Verification items for the finished model (mm, model axes). Face numbers are marked on the shaded views. A direction names the side the tool comes from. Give positions to 0.01 mm unless a question says otherwise; leave off trailing zeros. Order: outer loops, then holes, each group sorted by start corner. A loop starts at its lowest first (then second) coordinate and runs counter-clockwise, first axis right, second up.
(1) Scan lines: L1, parallel to X at y = 3, z = 0; L2, parallel to X at y = 21, z = 0; L3, parallel to X at y = 2.5, z = -6.35. Record each from-to range of solid material in increasing order.
(2) Mould release check, pull along X, two halves, no side actions. Record for the marked faces 3, 4, 5 and 6: pulls with the +X half, pulls with the -X half, needs draft (parallel to the pull), parting line crosses it, or undercut.
(3) Sectioned sample at C-C on x = 0. Record the cut outline in (y, z), plus the area to 3 significant figures.
(4) Sectioned sample at A-A on y = 36.5. Count the separate pieces of the cut face and the enclosed holes in it, plus the area to 3 significant figures.
(5) Access from +Z, -Z, +X, -X, +Y, -Y to the whole of each face (thin tool, end or side, straight path). Record for the marked faces 1 and 2.
(6) Gauge pin test, flat end, axial feed: pin 1 (2 mm diameter, centred on x = -2.5, z = 15.5, fed in from +Y). Record the tip position at first contact, or that the pin passes through.
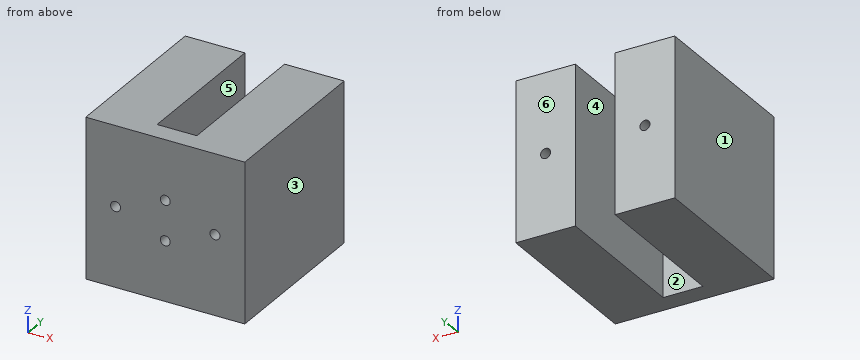
```python
from build123d import *

# Parameters (mm, degrees)
SKETCH1_W           = 50.8
SKETCH1_H           = 50.8
BOSS_EXTRUDE1_DEPTH = 6.35
SKETCH2_W           = 19.05
SKETCH2_H           = 50.8
BOSS_EXTRUDE2_DEPTH = 47.625
SKETCH3_R           = 1.5875
CUT_EXTRUDE1_DEPTH  = 60.652834174
SKETCH4_R           = 1.5875
CUT_EXTRUDE2_DEPTH  = 65.835334695


with BuildPart() as part:
    # Sketch1 → Boss-Extrude1 (new body)
    with BuildSketch(Plane(origin=(0, 0, 0), x_dir=(1, 0, 0), z_dir=(0, 1, 0))):
        Rectangle(SKETCH1_W, SKETCH1_H)
    extrude(amount=BOSS_EXTRUDE1_DEPTH)

    # Sketch2 → Boss-Extrude2 (add)
    with BuildSketch(Plane(origin=(0, 6.35, 0), x_dir=(1, 0, 0), z_dir=(0, 1, 0))):
        with Locations((-15.875, 0)):
            Rectangle(SKETCH2_W, SKETCH2_H)
        with Locations((15.875, 0)):
            Rectangle(SKETCH2_W, SKETCH2_H)
    extrude(amount=BOSS_EXTRUDE2_DEPTH)

    # Sketch3 → Cut-Extrude1 (cut, through all)
    with BuildSketch(Plane(origin=(0, 6.35, 0), x_dir=(1, 0, 0), z_dir=(0, 1, 0))):
        with Locations(Location((0, 6.35, 0), (0, 0, 270))):
            Circle(SKETCH3_R)
        with Locations(Location((0, -6.35, 0), (0, 0, 270))):
            Circle(SKETCH3_R)
    extrude(amount=-CUT_EXTRUDE1_DEPTH, mode=Mode.SUBTRACT)

    # Sketch4 → Cut-Extrude2 (cut, through all)
    with BuildSketch(Plane(origin=(0, 53.975, 0), x_dir=(1, 0, 0), z_dir=(0, 1, 0))):
        with Locations(Location((-15.875, 0, 0), (0, 0, 270))):
            Circle(SKETCH4_R)
        with Locations(Location((15.875, 0, 0), (0, 0, 270))):
            Circle(SKETCH4_R)
    extrude(amount=-CUT_EXTRUDE2_DEPTH, mode=Mode.SUBTRACT)


solid = part.part
```
Ans:
1. L1: x = -25.4 to -17.46, -14.29 to 14.29, 17.46 to 25.4
1. L2: x = -25.4 to -17.46, -14.29 to -6.35, 6.35 to 14.29, 17.46 to 25.4
1. L3: x = -25.4 to -1.59, 1.59 to 25.4
2. face 3: pulls with the +X half
2. face 4: undercut
2. face 5: undercut
2. face 6: needs draft
3. outline: (0, -25.4) - (6.35, -25.4) - (6.35, -7.94) - (0, -7.94) - close; (0, -4.76) - (6.35, -4.76) - (6.35, 4.76) - (0, 4.76) - close; (0, 7.94) - (6.35, 7.94) - (6.35, 25.4) - (0, 25.4) - close
3. area: 282 mm2
4. separate pieces: 2
4. enclosed holes: 2
4. area: 1,920 mm2
5. face 1: +Z, -Z, -X, +Y, -Y
5. face 2: +Z, -Z, +Y
6. pin 1: stops at y = 6.35
